Can you work these out from the model? Positions are in its coordinate system, mm. Face numbers are marked on the shaded views. A direction names the side the tool comes from. Coordinates: 2 decimals unless noted, no trailing zeros. Write each loop counter-clockwise with the first axis right and the second up, starting at its lowest first coordinate (ties: lowest second). Pieces come first, ordered by that corner, then holes. Notation, with made-up numbers: M -14.75,9 L 44.25,9 A14 cw 44.25,26 Z; hole C 4.25,59.25 d1. An arc over 180 degrees is marked long. Use one line per item in the form item = value. Start each with the question number.
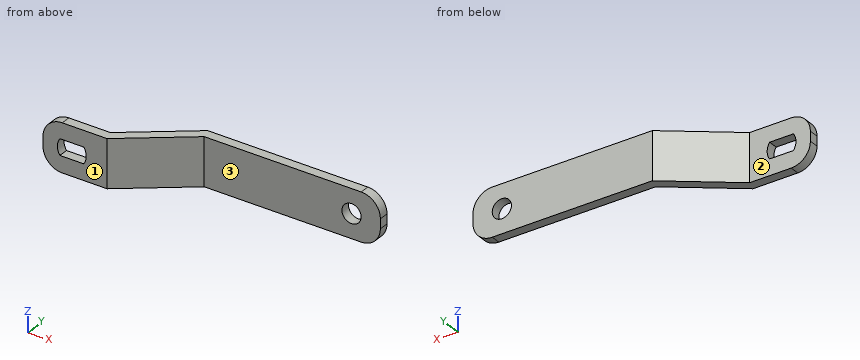
```python
from build123d import *

# Parameters (mm, degrees)
BOSS_EXTRU_1_DEPTH      = 15
ESQUISSE3_OUTSIDE_W     = 116.57
ESQUISSE3_OUTSIDE_H     = 36.57
ESQUISSE3_OUTSIDE_R     = 3
ENL_V_MAT_EXTRU_1_DEPTH = 19


with BuildPart() as part:
    # Esquisse1 → Boss.-Extru.1 (new body)
    with BuildSketch(Plane.XY):
        Polygon((0, 0), (20, 0), (40, 15), (95, 15), (95, 18), (39, 18), (19, 3), (0, 3), align=None)
    extrude(amount=BOSS_EXTRU_1_DEPTH)

    # Esquisse3 outside → Enlèv. mat.-Extru.1 (cut, through all)
    with BuildSketch(Plane(origin=(0, 18, 0), x_dir=(1, 0, 0), z_dir=(0, 1, 0))):
        with Locations((47.5, -7.5)):
            Rectangle(ESQUISSE3_OUTSIDE_W, ESQUISSE3_OUTSIDE_H)
        with BuildLine():
            Line((6, 0), (89, 0))
            ThreePointArc((89, 0), (93.242640687, -1.757359313), (95, -6))
            Line((95, -6), (95, -9))
            ThreePointArc((95, -9), (93.242640687, -13.242640687), (89, -15))
            Line((89, -15), (6, -15))
            ThreePointArc((6, -15), (1.757359313, -13.242640687), (0, -9))
            Line((0, -9), (0, -6))
            ThreePointArc((0, -6), (1.757359313, -1.757359313), (6, 0))
        make_face(mode=Mode.SUBTRACT)
        with Locations((86, -7.5)):
            Circle(ESQUISSE3_OUTSIDE_R)
        with BuildLine():
            Line((5.258342613, -5), (12.741657387, -5))
            ThreePointArc((12.741657387, -5), (13.5, -7.5), (12.741657387, -10))
            Line((12.741657387, -10), (5.258342613, -10))
            ThreePointArc((5.258342613, -10), (4.5, -7.5), (5.258342613, -5))
        make_face()
    extrude(amount=-ENL_V_MAT_EXTRU_1_DEPTH, mode=Mode.SUBTRACT)


solid = part.part
```
1) Suppose I cut it at C-C on x = 70. Please give me the cut outline in (y, z).
2) Suppose I cut it at B-B on x = 86. Please give me the cut outline in (y, z).
3) Will these pins go through, and if not, where does the flat tip stop? pin 1 Ø1 at (y, z) = (12, 3.5) entering from +X; pin 2 Ø4 at (y, z) = (7.5, 7) entering from +X; pin 3 Ø1.5 at (x, y) = (37, 10.5) entering from -Z; pin 4 Ø1.5 at (x, z) = (31.5, 5) entering from -Y.
4) Which directions (+Z, -Z, +X, -X, +Y, -Y) give clear straight access to the entire face, cutting with the end or side of a thin tool? Please do the marked faces 1, 2 and 3.
5) Please list where these lines run through material, in increasing order: line 1 (Z direction, x = 86, y = 16.85); line 2 (Y direction, x = 76, z = 13.25); line 3 (X direction, y = 17.1, z = 7.5).
6) Suppose I cut it at A-A on z = 7.5. Please give me the cut outline in (x, y).
7) Suppose I cut it at D-D on y = 10.25. Please give me the cut outline in (x, z), and give its area (3 significant figures).
Computed values:
q1.outline = M 15,0 L 18,0 L 18,15 L 15,15 Z
q2.outline = M 15,0 L 18,0 L 18,4.5 L 15,4.5 Z; M 15,10.5 L 18,10.5 L 18,15 L 15,15 Z
q3.pin_1 = 36.67
q3.pin_2 = 32.67
q3.pin_3 = through
q3.pin_4 = 8.06
q4.face_1 = +Z, -Z, +X, -X, -Y
q4.face_2 = +Z, -Z, -X, +Y
q4.face_3 = +Z, -Z, +X, -Y
q5.line_1 = 0 to 4.5, 10.5 to 15
q5.line_2 = 15 to 18
q5.line_3 = 37.8 to 83, 89 to 95
q6.outline = M 0,0 L 4.5,0 L 4.5,3 L 0,3 Z; M 13.5,0 L 20,0 L 40,15 L 83,15 L 83,18 L 39,18 L 19,3 L 13.5,3 Z; M 89,15 L 95,15 L 95,18 L 89,18 Z
q7.outline = M 28.67,0 L 33.67,0 L 33.67,15 L 28.67,15 Z
q7.area = 75.0 mm²
